Read the model definition and answer for the solid it produces. Units are mm, in the model's axes. A direction names the side the tool comes from. Give positions to 0.01 mm unless a question says otherwise; leave off trailing zeros. Loops run counter-clockwise (first coordinate to the right, second up) from the corner with the lowest first, then second, coordinate; pieces in that order, holes last. Notation, with made-up numbers: (50.25, 1) - (103.25, 1) arc R23 cw to (103.25, 22) - close; hole circle Ø4 at (22.25, 17). An arc over 180 degrees is marked (long way). Use a Markdown table: item, result. Add a question column.
Item 1: A cutting plane is placed at C-C (z = 53.5). Determine the outline of the cut face in (x, y).
Item 2: A cutting plane is placed at A-A (z = -18). Determine the outline of the cut face in (x, y).
Item 3: A cutting plane is placed at B-B (x = 17.5). Determine the outline of the cut face in (y, z), plus the area to 3 significant figures.
Item 4: For a pull along X with two mould halves and no side action, classify faces 1 (the face through (5.038, 1.479, -24.375)), 2 (the face through (-54, 1, 30.62)), 3 (the face through (-52.182, 1, 54)), 4 (the face through (54.818, 1, -58)) as +X half, -X half, draft (parallel to the pull), parting line (faces both ways), or undercut.
Item 5: Consider probe 1 along X at (y, z) = (1.05, 44); probe 2 along Z at (x, y) = (5, 1.45); probe 3 along Z at (x, y) = (4, 2.15). Determine where each line is inside the solid, lowest interval first. Write a range as [from, to].
Item 6: A cutting plane is placed at D-D (y = 0.45). Give the number of separate pieces and of enclosed holes in the cut face, plus the area to 3 significant figures.
Item 7: This flat-tipped pin is pushed along its axis until it touches: P1, Ø0.9, axis at y = 1, z = 18, coming from the -X side. Where does it stop, or does it pass through?
Item 8: Which of the six approach directions +Z, -Z, +X, -X, +Y, -Y give full straight-line access (tool end or side, diameter ignored) to faces 5 (the face through (4.818, 1, 59)), 6 (the face through (61.818, 1, -24)), 7 (the face through (-54, 1, 10.62))?
from build123d import *

# Parameters (mm, degrees)
SKETCH1_R           = 1.397
SKETCH1_R_2         = 5
BOSS_EXTRUDE1_DEPTH = 3


with BuildPart() as part:
    # Sketch1 → Boss-Extrude1 (new body)
    with BuildSketch(Plane(origin=(0, 0, 0), x_dir=(1, 0, 0), z_dir=(0, 1, 0))):
        Polygon((-45.181694993, 59.380211874), (-55.181694993, 59.380211874), (-55.181694993, 49.380211874), (-52.181694993, 49.380211874), (-52.181694993, 39.380211874), (-55.181694993, 39.380211874), (-55.181694993, 29.380211874), (-52.181694993, 29.380211874), (-52.181694993, 19.380211874), (-55.181694993, 19.380211874), (-55.181694993, 9.380211874), (-52.181694993, 9.380211874), (-52.181694993, -0.619788126), (-55.181694993, -0.619788126), (-55.181694993, -10.619788126), (-52.181694993, -10.619788126), (-52.181694993, -20.619788126), (-55.181694993, -20.619788126), (-55.181694993, -30.619788126), (-52.181694993, -30.619788126), (-52.181694993, -40.619788126), (-55.181694993, -40.619788126), (-55.181694993, -50.619788126), (-52.181694993, -50.619788126), (-52.181694993, -57.619788126), (-55.181694993, -57.619788126), (-55.181694993, -60.619788126), (-45.181694993, -60.619788126), (-45.181694993, -57.619788126), (-35.181694993, -57.619788126), (-35.181694993, -60.619788126), (-25.181694993, -60.619788126), (-25.181694993, -57.619788126), (-15.181694993, -57.619788126), (-15.181694993, -60.619788126), (-5.181694993, -60.619788126), (-5.181694993, -57.619788126), (4.818305007, -57.619788126), (4.818305007, -60.619788126), (14.818305007, -60.619788126), (14.818305007, -57.619788126), (24.818305007, -57.619788126), (24.818305007, -60.619788126), (34.818305007, -60.619788126), (34.818305007, -57.619788126), (44.818305007, -57.619788126), (44.818305007, -60.619788126), (54.818305007, -60.619788126), (54.818305007, -57.619788126), (61.818305007, -57.619788126), (61.818305007, -50.619788126), (64.818305007, -50.619788126), (64.818305007, -40.619788126), (61.818305007, -40.619788126), (61.818305007, -30.619788126), (64.818305007, -30.619788126), (64.818305007, -20.619788126), (61.818305007, -20.619788126), (61.818305007, -10.619788126), (64.818305007, -10.619788126), (64.818305007, -0.619788126), (61.818305007, -0.619788126), (61.818305007, 9.380211874), (64.818305007, 9.380211874), (64.818305007, 19.380211874), (61.818305007, 19.380211874), (61.818305007, 29.380211874), (64.818305007, 29.380211874), (64.818305007, 39.380211874), (61.818305007, 39.380211874), (61.818305007, 49.380211874), (64.818305007, 49.380211874), (64.818305007, 56.380211874), (54.818305007, 56.380211874), (54.818305007, 59.380211874), (44.818305007, 59.380211874), (44.818305007, 56.380211874), (34.818305007, 56.380211874), (34.818305007, 59.380211874), (24.818305007, 59.380211874), (24.818305007, 56.380211874), (14.818305007, 56.380211874), (14.818305007, 59.380211874), (4.818305007, 59.380211874), (4.818305007, 56.380211874), (-5.181694993, 56.380211874), (-5.181694993, 59.380211874), (-15.181694993, 59.380211874), (-15.181694993, 56.380211874), (-25.181694993, 56.380211874), (-25.181694993, 59.380211874), (-35.181694993, 59.380211874), (-35.181694993, 56.380211874), (-45.181694993, 56.380211874), align=None)
        with Locations(Location((-38.381694993, -43.779788126, 0), (0, 0, 270))):
            Circle(SKETCH1_R, mode=Mode.SUBTRACT)
        with Locations(Location((47.978305007, -43.779788126, 0), (0, 0, 270))):
            Circle(SKETCH1_R, mode=Mode.SUBTRACT)
        with Locations(Location((4.818305007, -20.619788126, 0), (0, 0, 270))):
            Circle(SKETCH1_R_2, mode=Mode.SUBTRACT)
        with Locations(Location((-38.381694993, 42.580211874, 0), (0, 0, 270))):
            Circle(SKETCH1_R, mode=Mode.SUBTRACT)
        with Locations(Location((4.818305007, 19.380211874, 0), (0, 0, 270))):
            Circle(SKETCH1_R_2, mode=Mode.SUBTRACT)
        with Locations(Location((47.978305007, 42.580211874, 0), (0, 0, 270))):
            Circle(SKETCH1_R, mode=Mode.SUBTRACT)
    extrude(amount=BOSS_EXTRUDE1_DEPTH)


solid = part.part
Geometry says:
| question | item | result |
|---|---|---|
| 1 | outline | (-52.18, 0) - (61.82, 0) - (61.82, 3) - (-52.18, 3) - close |
| 2 | outline | (-55.18, 0) - (0.01, 0) - (0.01, 3) - (-55.18, 3) - close; (9.62, 0) - (64.82, 0) - (64.82, 3) - (9.62, 3) - close |
| 3 | outline | (0, -56.38) - (3, -56.38) - (3, 57.62) - (0, 57.62) - close |
| 3 | area | 342 mm² |
| 4 | face 1 | undercut |
| 4 | face 2 | draft |
| 4 | face 3 | -X half |
| 4 | face 4 | +X half |
| 5 | probe 1 | [-55.18, -39.76], [-37, 46.6], [49.36, 64.82] |
| 5 | probe 2 | [-59.38, -24.38], [-14.38, 15.62], [25.62, 60.62] |
| 5 | probe 3 | [-56.38, -24.31], [-14.45, 15.69], [25.55, 57.62] |
| 6 | separate pieces | 1 |
| 6 | enclosed holes | 6 |
| 6 | area | 13,500 mm² |
| 7 | P1 | x = -52.18 |
| 8 | face 5 | +Z, +Y, -Y |
| 8 | face 6 | +X, +Y, -Y |
| 8 | face 7 | -X, +Y, -Y |
